Can you work these out from the model? Positions are in its coordinate system, mm. Give positions to 0.01 mm unless a question says otherwise; leave off trailing zeros. Return JSON: item names as keys, results as strings.
```python
from build123d import *

# Parameters (mm, degrees)
F0_W     = 355
F0_H     = 400
F0_R     = 36
F1_DEPTH = 3
F2_R     = 2
F3_DEPTH = 3
F4_R     = 6
F4_R_2   = 2.5
F5_DEPTH = 3


with BuildPart() as f1:
    # F0 (on Front) → F1 (new body)
    with BuildSketch(Plane.XZ):
        with Locations((177.5, 200)):
            Rectangle(F0_W, F0_H)
        with Locations((50, 242.5)):
            Circle(F0_R, mode=Mode.SUBTRACT)
        with Locations((135, 242.5)):
            Circle(F0_R, mode=Mode.SUBTRACT)
        with Locations((50, 327.5)):
            Circle(F0_R, mode=Mode.SUBTRACT)
        with Locations((135, 327.5)):
            Circle(F0_R, mode=Mode.SUBTRACT)
        with Locations((220, 242.5)):
            Circle(F0_R, mode=Mode.SUBTRACT)
        with Locations((305, 242.5)):
            Circle(F0_R, mode=Mode.SUBTRACT)
        with Locations((220, 327.5)):
            Circle(F0_R, mode=Mode.SUBTRACT)
        with Locations((305, 327.5)):
            Circle(F0_R, mode=Mode.SUBTRACT)
    extrude(amount=-F1_DEPTH)

    # F2 (on face) → F3 (cut)
    with BuildSketch(Plane.XZ):
        with Locations((20, 357.5)):
            Circle(F2_R)
        with Locations((80, 357.5)):
            Circle(F2_R)
        with Locations((80, 297.5)):
            Circle(F2_R)
        with Locations((20, 297.5)):
            Circle(F2_R)
        with Locations((80, 272.5)):
            Circle(F2_R)
        with Locations((80, 212.5)):
            Circle(F2_R)
        with Locations((20, 212.5)):
            Circle(F2_R)
        with Locations((20, 272.5)):
            Circle(F2_R)
        with Locations((165, 357.5)):
            Circle(F2_R)
        with Locations((165, 297.5)):
            Circle(F2_R)
        with Locations((105, 297.5)):
            Circle(F2_R)
        with Locations((105, 357.5)):
            Circle(F2_R)
        with Locations((165, 272.5)):
            Circle(F2_R)
        with Locations((165, 212.5)):
            Circle(F2_R)
        with Locations((105, 212.5)):
            Circle(F2_R)
        with Locations((105, 272.5)):
            Circle(F2_R)
        with Locations((250, 357.5)):
            Circle(F2_R)
        with Locations((250, 297.5)):
            Circle(F2_R)
        with Locations((190, 297.5)):
            Circle(F2_R)
        with Locations((190, 357.5)):
            Circle(F2_R)
        with Locations((250, 272.5)):
            Circle(F2_R)
        with Locations((250, 212.5)):
            Circle(F2_R)
        with Locations((190, 212.5)):
            Circle(F2_R)
        with Locations((190, 272.5)):
            Circle(F2_R)
        with Locations((335, 357.5)):
            Circle(F2_R)
        with Locations((335, 297.5)):
            Circle(F2_R)
        with Locations((275, 297.5)):
            Circle(F2_R)
        with Locations((275, 357.5)):
            Circle(F2_R)
        with Locations((335, 272.5)):
            Circle(F2_R)
        with Locations((335, 212.5)):
            Circle(F2_R)
        with Locations((275, 212.5)):
            Circle(F2_R)
        with Locations((275, 272.5)):
            Circle(F2_R)
    extrude(amount=-F3_DEPTH, mode=Mode.SUBTRACT)

    # F4 (on face) → F5 (cut)
    with BuildSketch(Plane.XZ):
        with Locations((35, 91)):
            Circle(F4_R)
        with Locations((55, 91)):
            Circle(F4_R)
        with Locations((75, 91)):
            Circle(F4_R)
        with Locations((106, 55)):
            Circle(F4_R)
        with Locations((126, 55)):
            Circle(F4_R)
        with Locations((146, 55)):
            Circle(F4_R)
        with Locations((41, 30)):
            Circle(F4_R)
        with Locations((83.710723, 20)):
            Circle(F4_R)
        with Locations((108.710723, 20)):
            Circle(F4_R)
        with Locations((133.710723, 20)):
            Circle(F4_R)
        with Locations((158.710723, 20)):
            Circle(F4_R)
        with Locations((183.710723, 20)):
            Circle(F4_R)
        with Locations((208.710723, 20)):
            Circle(F4_R)
        with Locations((233.710723, 20)):
            Circle(F4_R)
        with Locations((195, 60)):
            Circle(F4_R)
        with Locations((220, 60)):
            Circle(F4_R)
        with Locations((185, 385)):
            Circle(F4_R)
        with Locations((210, 385)):
            Circle(F4_R)
        with Locations((235, 385)):
            Circle(F4_R)
        with Locations((260, 385)):
            Circle(F4_R)
        with Locations((285, 385)):
            Circle(F4_R)
        with Locations((320, 380)):
            Circle(F4_R_2)
        with Locations((51.772643, 382.141024)):
            Circle(F4_R_2)
    extrude(amount=-F5_DEPTH, mode=Mode.SUBTRACT)


solid = f1.part
```
1. For pin 1 Ø11 at (x, z) = (55, 91) entering from +Y, with a flat end and sliding along its axis, tell me the tip position at first contact or that it passes through.
Checks:
{"pin 1": "through"}
2. Thinking about a two-plate mould opening in Z: for faces 1 (the face through (127.196, 1.479, 292.356)), 2 (the face through (175, 0, 203)), which applies, +Z half, -Z half, draft (parallel to the pull), parting line (faces both ways), or undercut?
Checks:
{"face 1": "undercut", "face 2": "draft"}
3. Suppose I cut it at A-A (y = 1.45). State how many separate pieces and enclosed holes the cut face has, plus the area to 3 significant figures.
Checks:
{"separate pieces": "1", "enclosed holes": "63", "area": "107,000 mm^2"}
4. If I drill on L1, parallel to Z at x = 327.5, y = 0.2; L2, parallel to X at y = 1.05, z = 385; L3, parallel to Z at x = 236, y = 2.15, over which ranges is the centre line in solid material (lowest first)? Write a range as [from, to].
Checks:
{"L1": "[0, 214.4], [270.6, 299.4], [355.6, 400]", "L2": "[0, 179], [191, 204], [216, 229], [241, 254], [266, 279], [291, 355]", "L3": "[0, 14.45], [25.55, 210.25], [274.75, 295.25], [359.75, 379.08], [390.92, 400]"}
